Check sheet for the drawn part. Datum: minimum x, y, z corner. Units: mm. A direction names the side the tool comes from. Give positions to 0.01 mm unless a question says otherwise; leave off trailing zeros. Write each loop counter-clockwise with the first axis right and the second up, starting at its lowest first coordinate (ties: lowest second). Pieces come first, ordered by that corner, then holes. Notation, with made-up numbers: (23, -18) - (34, -18) arc R26 ccw to (34, 17) - close; hole circle Ø9 at (-22.75, 80.25). An arc over 180 degrees is marked (long way). Answer as a JSON object with one key per item and string values. Group by question number.
Item 1: Sectioned sample at C-C, the plane z = 4. Record the boundary of the cut face in (x, y).
Item 2: Sectioned sample at D-D, the plane y = 3.5. Record the boundary of the cut face in (x, z), and give its area (3 significant figures).
Item 3: Scan lines: line 1 along X through (y, z) = (10.25, 19); line 2 along Y through (x, z) = (5.5, 20); line 3 along X through (y, z) = (7.75, 20.5). Record each from-to range of solid material in increasing order. Write a range as [from, to].
Item 4: Tool access check on the marked faces 4, 5, 6 and 7. Record the directions out of +Z, -Z, +X, -X, +Y, -Y that give a thin tool (end or side, any length) a straight path to the whole face; none if there is none.
Item 5: Go/stop test with flat-tipped pins: pin 1 (9 mm diameter, centred on y = 7.5, z = 17.5, fed in from +X); pin 2 (6.5 mm diameter, centred on x = 52.5, z = 5.5, fed in from +Y); pin 3 (0.6 mm diameter, centred on y = 6.5, z = 5.5, fed in from -X). Record where each tip stops, or that it passes through.
Item 6: Sectioned sample at B-B, the plane y = 14. Record the boundary of the cut face in (x, z).
Item 7: Draft check along Z on the marked faces 1, 2 and 3. Enter one of: +Z half, -Z half, draft (parallel to the pull), parting line (faces both ways), or undercut.
Item 8: Sectioned sample at A-A, the plane z = 10.75. Record the boundary of the cut face in (x, y).
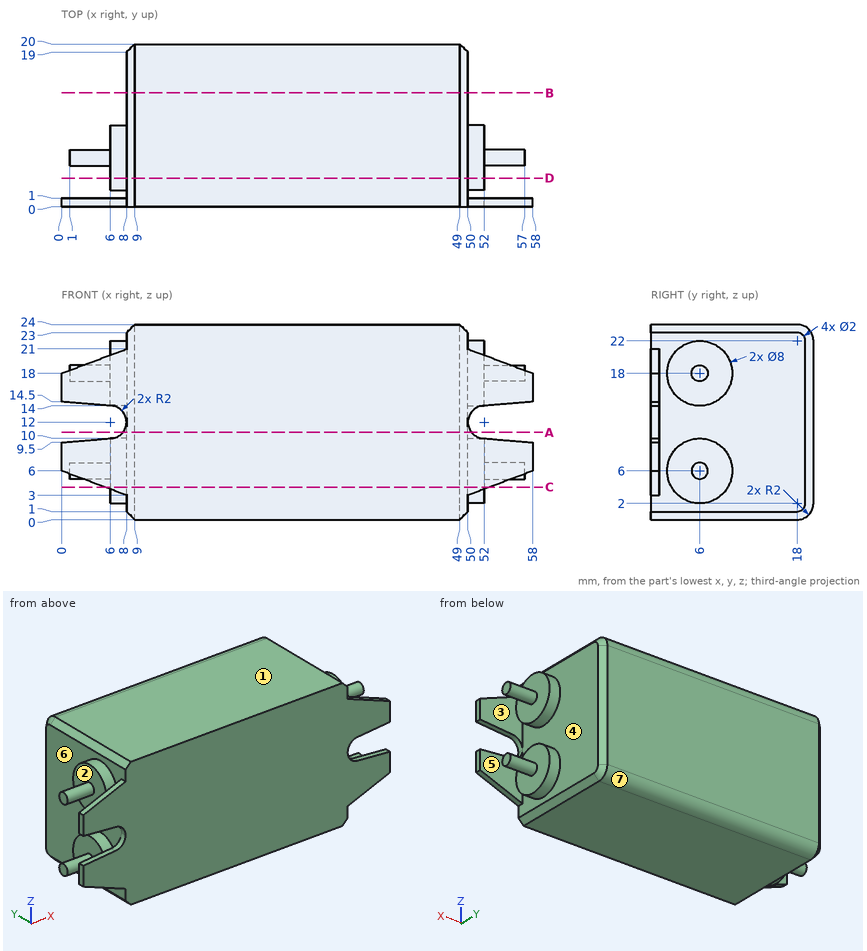
Geometry check:
{
 "1": {"outline": "(5.33, 0) - (52.67, 0) - (52.67, 1) - (50, 1) - (50, 2.54) - (52, 2.54) - (52, 9.46) - (50, 9.46) - (50, 19) - (49, 20) - (9, 20) - (8, 19) - (8, 9.46) - (6, 9.46) - (6, 2.54) - (8, 2.54) - (8, 1) - (5.33, 1) - close"},
 "2": {"outline": "(6, 2.88) - (8, 2.88) - (8, 1) - (9, 0) - (49, 0) - (50, 1) - (50, 2.88) - (52, 2.88) - (52, 9.12) - (50, 9.12) - (50, 14.88) - (52, 14.88) - (52, 21.12) - (50, 21.12) - (50, 23) - (49, 24) - (9, 24) - (8, 23) - (8, 21.12) - (6, 21.12) - (6, 14.88) - (8, 14.88) - (8, 9.12) - (6, 9.12) - close", "area": "1,060 mm^2"},
 "3": {"line 1": "[8, 50]", "line 2": "[0, 1]", "line 3": "[6, 52]"},
 "4": {"face 4": "+X", "face 5": "+Z, -Z, +X", "face 6": "-X", "face 7": "-Z, +X, -X, +Y"},
 "5": {"pin 1": "x = 57", "pin 2": "y = 19.75", "pin 3": "x = 1"},
 "6": {"outline": "(8, 1) - (9, 0) - (49, 0) - (50, 1) - (50, 23) - (49, 24) - (9, 24) - (8, 23) - close"},
 "7": {"face 1": "+Z half", "face 2": "undercut", "face 3": "draft"},
 "8": {"outline": "(7.56, 0) - (50.44, 0) - (50.44, 1) - (50, 1) - (50, 19) - (49, 20) - (9, 20) - (8, 19) - (8, 1) - (7.56, 1) - close"}
}
